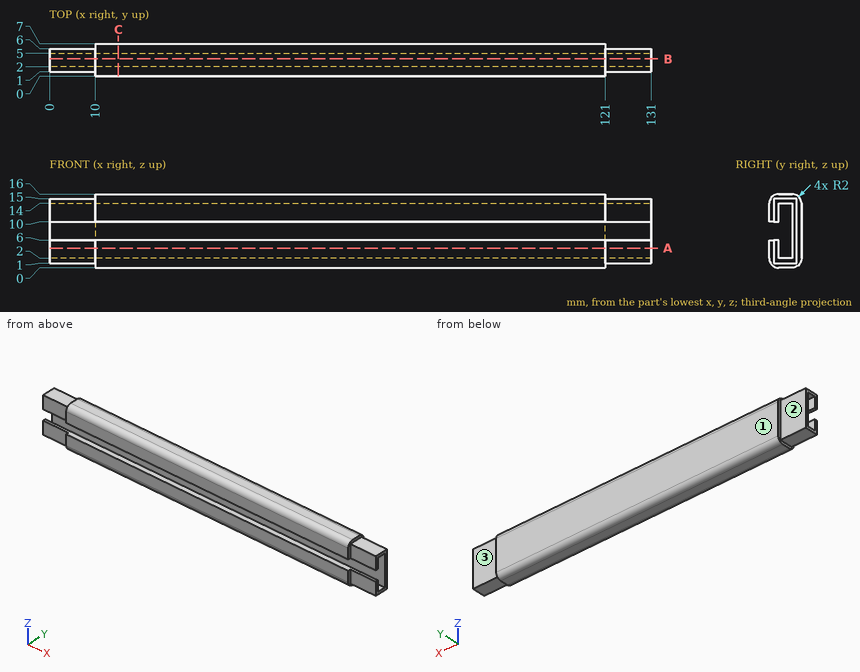
Geometry: see drawing. Coordinates: mm, zero at the bounding-box minimum. A direction names the side the tool comes from. Give positions to 0.01 mm unless a question says otherwise; leave off trailing zeros. Order: outer loops, then holes, each group sorted by start corner. A loop starts at its lowest first (then second) coordinate and runs counter-clockwise, first axis right, second up. Notation, with made-up numbers: (55, 79.25) - (106, 79.25) arc R21 ccw to (106, 99.25) - close; hole circle Ø6 at (78, 3.5). An arc over 180 degrees is marked (long way). One line per item, written item: value.
1. Pin query (flat end, axial travel): pin 1 Ø3 at (y, z) = (2.5, 8) entering from +X; pin 2 Ø4 at (x, z) = (126.5, 3.5) entering from -Y; pin 3 Ø2.5 at (x, y) = (2.5, 3.5) entering from +Z; pin 4 Ø1.6 at (x, y) = (51, 1) entering from -Z. Return the tip coordinate at first contact, or that it passes through.
Determined:
pin 1: through
pin 2: y = 1
pin 3: z = 15
pin 4: z = 0.01
2. Cut plane B-B, the plane y = 3.75. Output: boundary loops of the cut face in (x, z), and give its area (3 significant figures).
Determined:
outline: (0, 1) - (10, 1) - (10, 0) - (121, 0) - (121, 1) - (131, 1) - (131, 2) - (0, 2) - close; (0, 14) - (131, 14) - (131, 15) - (121, 15) - (121, 16) - (10, 16) - (10, 15) - (0, 15) - close
area: 484 mm2
3. Line query: probe 1 along Y at (x, z) = (95.5, 12); probe 2 along Z at (x, y) = (8, 4.5); probe 3 along Z at (x, y) = (27.5, 2.5). Output: solid intervals per line, ascending.
Determined:
probe 1: 0 to 2, 5 to 7
probe 2: 1 to 2, 14 to 15
probe 3: 0 to 2, 14 to 16
4. Cut plane A-A, the plane z = 4.25. Output: boundary loops of the cut face in (x, y).
Determined:
outline: (0, 1) - (10, 1) - (10, 0) - (121, 0) - (121, 1) - (131, 1) - (131, 2) - (0, 2) - close; (0, 5) - (131, 5) - (131, 6) - (121, 6) - (121, 7) - (10, 7) - (10, 6) - (0, 6) - close
5. Cut plane C-C, the plane x = 15. Output: boundary loops of the cut face in (y, z), and give its area (3 significant figures).
Determined:
outline: (0, 2) arc R2 ccw to (2, 0) - (5, 0) arc R2 ccw to (7, 2) - (7, 14) arc R2 ccw to (5, 16) - (2, 16) arc R2 ccw to (0, 14) - (0, 10) - (2, 10) - (2, 14) - (5, 14) - (5, 2) - (2, 2) - (2, 6) - (0, 6) - close
area: 64.6 mm2
6. Reachability of the marked faces 1, 2 and 3 from +Z, -Z, +X, -X, +Y, -Y: full face, straight path, thin tool, end or side. Return the list, or none.
Determined:
face 1: +Z, -Z, +X, -X, +Y
face 2: +Z, -Z, -X, +Y
face 3: +Z, -Z, +X, +Y
